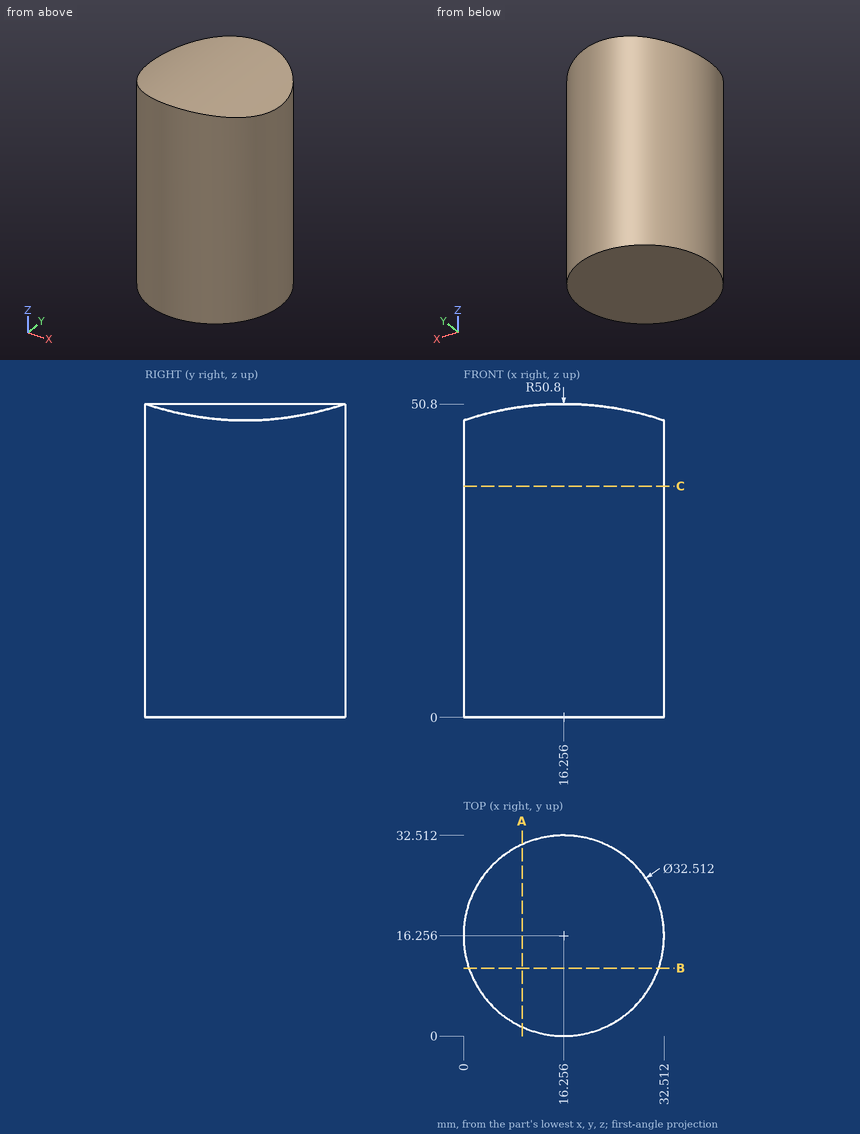
Print and shaded views of the part. All mm, measured from the part's lowest x, y and z. Round coordinates to 2 decimals unless told otherwise and drop trailing zeros. Loops run counter-clockwise (first coordinate to the right, second up) from the corner with the lowest first, then second, coordinate; pieces in that order, holes last. Notation, with made-up numbers: (1.25, 88.25) -> (51.25, 88.25) arc R17 ccw to (51.25, 94.25) -> close; hole circle Ø9 at (59, 26). An arc over 180 degrees is marked (long way). Use CSV: the item, a comma, the result in double quotes. Start each with the question number.
1) Wall check: L1, parallel to X at y = 16, z = 14.5; L2, parallel to X at y = 7, z = 20.5; L3, parallel to Z at x = 9, y = 18. Give the ranges that are in metal, low to high. Write a range as [from, to].
2) Cut at A-A, the plane x = 9.5. Write the cut outline in (y, z).
3) Cut at C-C, the plane z = 37.5. Write the cut outline in (x, y).
4) Drop flat-ended pins along their axis: P1, Ø1, axis at x = 21, z = 44, coming from the -Y side; P2, Ø10, axis at y = 27.5, z = 21.5, coming from the -X side; P3, Ø4, axis at x = 4.5, y = 5, coming from the -Z side; P4, Ø10, axis at x = 11, z = 6, coming from the +Y side. Give the stop position or say it passes through.
5) Cut at B-B, the plane y = 11. Write the cut outline in (x, z).
Determined:
1,L1,"x = [0, 32.51]"
1,L2,"x = [2.89, 29.62]"
1,L3,"z = [0, 50.28]"
2,outline,"(1.47, 0) -> (31.04, 0) -> (31.04, 50.35) -> (1.47, 50.35) -> close"
3,outline,"circle Ø32.51 at (16.26, 16.26)"
4,P1,"stops at y = 0.56"
4,P2,"stops at x = 1.25"
4,P3,"stops at z = 0"
4,P4,"stops at y = 32.51"
5,outline,"(0.87, 0) -> (31.64, 0) -> (31.64, 48.41) arc R50.8 ccw to (0.87, 48.41) -> close"
